Build history of the part. All positions in model axes, mm. Give positions to 0.01 mm unless a question says otherwise; leave off trailing zeros. Write each loop counter-clockwise with the first axis right and the second up, starting at its lowest first coordinate (ties: lowest second). Pieces come first, ordered by that corner, then holes. Notation, with made-up numbers: (62, -24) -> (118, -24) arc R20 cw to (118, -20) -> close; hole circle Ø4 at (60, 22). An arc over 180 degrees is marked (long way). Put each result on its own line as item: value.
from build123d import *

# Parameters (mm, degrees)
F0_W          = 50.8
F0_H          = 12.7
F1_DEPTH      = 50.8
F2_R          = 2.5527
F2_R_2        = 4.7625
F3_DEPTH      = 12.701
F4_W          = 50.8
F4_H          = 50.8
F4_R          = 4.7625
F4_R_2        = 9.525
F5_DEPTH      = 12.7
F6_W          = 50.8
F6_H          = 50.8
F6_R          = 4.7625
F6_R_2        = 3.175
F7_DEPTH      = 6.35
F8_R          = 2.8575
F9_DEPTH      = 38.1
F9_DEPTH_BACK = 15.875
F10_R         = 19.05
F11_DEPTH     = 9.525
F12_R         = 2.8575
F13_DEPTH     = 1.5875


with BuildPart() as f1:
    # F0 (on Front) → F1 (new body)
    with BuildSketch(Plane.XZ):
        with Locations((0, 6.35)):
            Rectangle(F0_W, F0_H)
    extrude(amount=F1_DEPTH)

    # F2 (on face) → F3 (cut, through all)
    with BuildSketch(Plane.XY.offset(12.7)):
        with Locations((-12.7, -12.7)):
            Circle(F2_R)
        with Locations((-12.7, -38.1)):
            Circle(F2_R)
        with Locations((12.7, -38.1)):
            Circle(F2_R)
        with Locations((12.7, -12.7)):
            Circle(F2_R)
        with Locations((0, -25.4)):
            Circle(F2_R_2)
    extrude(amount=-F3_DEPTH, mode=Mode.SUBTRACT)


with BuildPart() as f5:
    # F4 (on face) → F5 (new body)
    with BuildSketch(Plane.XY.offset(12.7)):
        with Locations((0, -25.4)):
            Rectangle(F4_W, F4_H)
        with Locations((-12.7, -38.1)):
            Circle(F4_R, mode=Mode.SUBTRACT)
        with Locations((0, -25.4)):
            Circle(F4_R_2, mode=Mode.SUBTRACT)
        with Locations((12.7, -38.1)):
            Circle(F4_R, mode=Mode.SUBTRACT)
        with Locations((-12.7, -12.7)):
            Circle(F4_R, mode=Mode.SUBTRACT)
        with Locations((12.7, -12.7)):
            Circle(F4_R, mode=Mode.SUBTRACT)
    extrude(amount=F5_DEPTH)

    # F6 (on face) → F7 (join)
    with BuildSketch(Plane.XY.offset(25.4)):
        with Locations((0, -25.4)):
            Rectangle(F6_W, F6_H)
        with Locations((-12.7, -38.1)):
            Circle(F6_R, mode=Mode.SUBTRACT)
        with Locations((0, -25.4)):
            Circle(F6_R_2, mode=Mode.SUBTRACT)
        with Locations((12.7, -38.1)):
            Circle(F6_R, mode=Mode.SUBTRACT)
        with Locations((-12.7, -12.7)):
            Circle(F6_R, mode=Mode.SUBTRACT)
        with Locations((12.7, -12.7)):
            Circle(F6_R, mode=Mode.SUBTRACT)
    extrude(amount=F7_DEPTH)


with BuildPart() as f9:
    # F8 (on face) → F9 (new body, two sides)
    with BuildSketch(Plane.XY.offset(31.75)) as f9_sk:
        with Locations((0, -25.4)):
            Circle(F8_R)
    extrude(amount=-F9_DEPTH)
    extrude(f9_sk.sketch, amount=-F9_DEPTH_BACK)

    # F10 (on face) → F11 (join)
    with BuildSketch(Plane.XY.offset(47.625)):
        with Locations((0, -25.4)):
            Circle(F10_R)
    extrude(amount=F11_DEPTH)


with BuildPart() as f13:
    # F12 (on face) → F13 (new body)
    with BuildSketch(Plane.XY.offset(12.7)):
        Polygon((4.7625, -28.149631), (4.7625, -22.650369), (0, -19.900739), (-4.7625, -22.650369), (-4.7625, -28.149631), (0, -30.899261), align=None)
        with Locations((0, -25.4)):
            Circle(F12_R, mode=Mode.SUBTRACT)
    extrude(amount=F13_DEPTH)


solid = f1.part
1) Pin check, flat tip, straight feed: pin 1 (3 mm diameter, centred on x = 3, y = -26.5, fed in from +Z). Stop position of the tip, or through.
Filled sheet:
pin 1: through
2) Slice it at B-B (y = -38.1). Write the cut outline in (x, z).
Filled sheet:
outline: (-25.4, 0) -> (-15.25, 0) -> (-15.25, 12.7) -> (-25.4, 12.7) -> close; (-10.15, 0) -> (10.15, 0) -> (10.15, 12.7) -> (-10.15, 12.7) -> close; (15.25, 0) -> (25.4, 0) -> (25.4, 12.7) -> (15.25, 12.7) -> close
3) Wall check: L1, parallel to Y at x = 12.7, z = 3.75; L2, parallel to Y at x = -14.5, z = 11.5; L3, parallel to Y at x = 0, z = 11. Give the ranges that are in metal, low to high.
Filled sheet:
L1: -50.8 to -40.65, -35.55 to -15.25, -10.15 to 0
L2: -50.8 to -39.91, -36.29 to -14.51, -10.89 to 0
L3: -50.8 to -30.16, -20.64 to 0
4) Slice it at C-C (x = 0). Write the cut outline in (y, z), plus the area to 3 significant figures.
Filled sheet:
outline: (-50.8, 0) -> (-30.16, 0) -> (-30.16, 12.7) -> (-50.8, 12.7) -> close; (-20.64, 0) -> (0, 0) -> (0, 12.7) -> (-20.64, 12.7) -> close
area: 524 mm2
5) Slice it at A-A (y = -25.4). Write the cut outline in (x, z).
Filled sheet:
outline: (-25.4, 0) -> (-4.76, 0) -> (-4.76, 12.7) -> (-25.4, 12.7) -> close; (4.76, 0) -> (25.4, 0) -> (25.4, 12.7) -> (4.76, 12.7) -> close
6) Pull direction X, two halves, no side cores. Call faces 1 (the cylindrical face through (14.072, -35.948, 6.439)), 2 (the cylindrical face through (-13.03, -35.57, 6.44)), 3 (the flat face through (-25.4, -25, 6)), 4 (the flat face through (5, -25, 12.7)): released by +X, released by -X, zero draft, split by the parting line, or undercut.
Filled sheet:
face 1: undercut
face 2: undercut
face 3: released by -X
face 4: zero draft
7) Slice it at D-D (z = 11). Write the cut outline in (x, y) (1 decimal), plus the area to 3 significant figures.
Filled sheet:
outline: (-25.4, -50.8) -> (25.4, -50.8) -> (25.4, 0) -> (-25.4, 0) -> close; hole circle Ø5.1 at (-12.7, -38.1); hole circle Ø5.1 at (-12.7, -12.7); hole circle Ø9.5 at (0, -25.4); hole circle Ø5.1 at (12.7, -38.1); hole circle Ø5.1 at (12.7, -12.7)
area: 2,430 mm2
